Source: CAD feature listing. Evaluate the final solid. Frame: model axes, mm. Face numbers are marked on the shaded views. A direction names the side the tool comes from. Coordinates: 2 decimals unless noted, no trailing zeros. Order: outer loops, then holes, each group sorted by start corner. A loop starts at its lowest first (then second) coordinate and runs counter-clockwise, first axis right, second up.
```python
from build123d import *

# Parameters (mm, degrees)
SKETCH2_R               = 2.4892
BOSS_EXTRUDE3_DEPTH     = 9.525
SKETCH3_R               = 2.4892
BOSS_EXTRUDE4_DEPTH     = 9.525
SKETCH4_W               = 12.7
SKETCH4_H               = 1.27
BOSS_EXTRUDE5_DEPTH     = 9.525
SKETCH5_R               = 2.4892
CUT_EXTRUDE1_DEPTH      = 1
CUT_EXTRUDE1_DEPTH_BACK = 10.525
BOSS_EXTRUDE7_DEPTH     = 9.525


with BuildPart() as part:
    # Sketch2 → Boss-Extrude3 (new body)
    with BuildSketch(Plane(origin=(0, 0, 0), x_dir=(1, 0, 0), z_dir=(0, 1, 0))):
        with Locations((6.35, 6.35)):
            Circle(SKETCH2_R)
    extrude(amount=BOSS_EXTRUDE3_DEPTH)

    # Sketch3 → Boss-Extrude4 (add)
    with BuildSketch(Plane(origin=(0, 9.525, 0), x_dir=(1, 0, 0), z_dir=(0, 1, 0))):
        Polygon((9.525, 12.7), (3.175, 12.7), (3.175, 6.985), (0.975295474, 8.255), (0.975295474, 1.905), (3.175, 3.175), (3.175, 0), (9.525, 0), align=None)
        with Locations((6.35, 6.35)):
            Circle(SKETCH3_R, mode=Mode.SUBTRACT)
        Polygon((-3.175, 12.7), (-3.175, 6.35), (3.175, 12.7), align=None)
    extrude(amount=-BOSS_EXTRUDE4_DEPTH)

    # Sketch4 → Boss-Extrude5 (add)
    with BuildSketch(Plane(origin=(0, 9.525, 0), x_dir=(1, 0, 0), z_dir=(0, 1, 0))):
        with Locations((3.175, 13.335)):
            Rectangle(SKETCH4_W, SKETCH4_H)
    extrude(amount=-BOSS_EXTRUDE5_DEPTH)

    # Sketch5 → Cut-Extrude1 (cut, two sides)
    with BuildSketch(Plane(origin=(0, 9.525, 0), x_dir=(1, 0, 0), z_dir=(0, 1, 0))) as cut_extrude1_sk:
        with Locations((6.35, 6.35)):
            Circle(SKETCH5_R)
    extrude(amount=CUT_EXTRUDE1_DEPTH, mode=Mode.SUBTRACT)
    extrude(cut_extrude1_sk.sketch, amount=-CUT_EXTRUDE1_DEPTH_BACK, mode=Mode.SUBTRACT)

    # Sketch7 → Boss-Extrude7 (add)
    with BuildSketch(Plane(origin=(0, 9.525, 0), x_dir=(1, 0, 0), z_dir=(0, 1, 0))):
        Polygon((9.525, 13.97), (9.525, 17.212483646), (-3.175, 21.571193519), (-3.175, 13.97), align=None)
    extrude(amount=-BOSS_EXTRUDE7_DEPTH)


solid = part.part
```
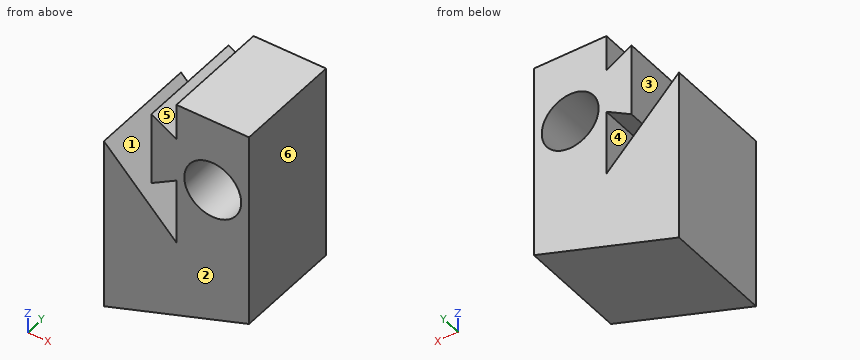
1. Section query A-A on y = 8. Return loops of the section in (x, z) (3 decimals), plus the area to 3 significant figures.
Findings:
outline: (-3.175, -21.571) - (9.525, -17.212) - (9.525, 0) - (3.175, 0) - (3.175, -3.175) - (0.975, -1.905) - (0.975, -8.255) - (3.175, -6.985) - (3.175, -12.7) - (-3.175, -6.35) - close; hole circle Ø4.978 at (6.35, -6.35)
area: 178 mm2
2. Draft query along Z for the marked faces 4, 5 and 6. Return one class per face: released by +Z, released by -Z, zero draft, split by the parting line, or undercut.
Findings:
face 4: undercut
face 5: released by +Z
face 6: zero draft
3. Section query B-B on x = 6.35. Return loops of the section in (y, z) (3 decimals), plus the area to 3 significant figures.
Findings:
outline: (0, -18.302) - (9.525, -18.302) - (9.525, -8.839) - (0, -8.839) - close; (0, -3.861) - (9.525, -3.861) - (9.525, 0) - (0, 0) - close
area: 127 mm2
4. Section query D-D on z = -1.5. Return loops of the section in (x, y) (3 decimals), plus the area to 3 significant figures.
Findings:
outline: (3.175, 0) - (9.525, 0) - (9.525, 9.525) - (3.175, 9.525) - close
area: 60.5 mm2
5. Section query C-C on z = -9.25. Return loops of the section in (x, y) (3 decimals).
Findings:
outline: (-3.175, 0) - (-0.275, 0) - (-0.275, 9.525) - (-3.175, 9.525) - close; (3.175, 0) - (9.525, 0) - (9.525, 9.525) - (3.175, 9.525) - close
6. Access query for the marked faces 1, 2 and 3. Directions: +Z, -Z, +X, -X, +Y, -Y. A direction counts if a zero-diameter tool reaches every point of the face in a straight line with its end or side. Return the directions, or none.
Findings:
face 1: +Y, -Y
face 2: +Z, -Z, +X, -X, -Y
face 3: +Z, +Y, -Y
7. Pin query (flat end, axial travel): P1, Ø1.6, axis at y = 3, z = -2, coming from the -X side; P2, Ø5, axis at y = 4.5, z = -5.5, coming from the -X side (3 decimals). Return the tip coordinate at first contact, or that it passes through.
Findings:
P1: stops at x = 0.98
P2: stops at x = -3.175
8. Ray query, line 1 (X direction, y = 7, z = -3.5) (3 decimals); line 2 (Z direction, x = 6.75, y = 2.25); line 3 (Z direction, x = 2, y = 6.25) (3 decimals). Return the intervals inside material, ascending.
Findings:
line 1: x = 0.975 to 9.525
line 2: z = -18.16 to -8.81, -3.89 to 0
line 3: z = -19.795 to -11.525, -7.663 to -2.497
